Autodesk Inventor part; units mm, degrees
ref_plane "YZ Plane" through (0, 0, 0) normal (1, 0, 0) x (0, 1, 0)
ref_plane "XZ Plane" through (0, 0, 0) normal (0, 1, 0) x (-1, 0, 0)
ref_plane "XY Plane" through (0, 0, 0) normal (0, 0, 1) x (1, 0, 0)
sketch "Эскиз1" plane through (0, 0, 0) normal (0, 0, 1) x (1, 0, 0)
  line L0 (0, 0) -> (0, 13)
  line L1 (0, 13) -> (16.5, 13)
  line L2 (16.5, 13) -> (16.5, 10)
  line L3 (16.5, 10) -> (14.5, 10)
  line L4 (14.5, 10) -> (14.5, 3)
  line L5 (14.5, 3) -> (13.5, 3)
  line L6 (13.5, 3) -> (13.5, 0)
  line L7 (13.5, 0) -> (0, 0)
  dimension "d0" = 13
  dimension "d1" = 16.5
  dimension "d2" = 3
  dimension "d3" = 2
  dimension "d4" = 7
  dimension "d5" = 1
revolve "Вращение1" add sketch "Эскиз1" angle 360 about axis through (0, 0, 0) along (0, 1, 0)
sketch "Эскиз2" plane through (0, 13, 0) normal (0, 1, 0) x (1, 0, 0)
  circle A0 centre (0, 0) radius 3
  line L0 (-5, -7) -> (5, -7)
  line L1 (7, -5) -> (7, 5)
  line L2 (5, 7) -> (-5, 7)
  line L3 (-7, 5) -> (-7, -5)
  line L4 (-7, -7) -> (7, 7) construction
  line L5 (7, -7) -> (-7, 7) construction
  arc A1 (-7, -5) -> (-5, -7) centre (-5, -5) ccw
  arc A2 (5, -7) -> (7, -5) centre (5, -5) ccw
  arc A3 (7, 5) -> (5, 7) centre (5, 5) ccw
  arc A4 (-5, 7) -> (-7, 5) centre (-5, 5) ccw
  dimension "d7" = 6
  dimension "d8" = 14
  dimension "d9" = 14
  dimension "d10" = 2
extrude "Выдавливание1" cut sketch "Эскиз2" against normal blind 24 contours A0
extrude "Выдавливание2" add sketch "Эскиз2" along normal blind 5
chamfer "Фаска1" distance 2 angle 45 8 edges at (0, 13, 7) (-6.4142, 13, 6.4142) (-7, 13, 0) (-6.4142, 13, -6.4142) (0, 13, -7) (6.4142, 13, -6.4142) (7, 13, 0) (6.4142, 13, 6.4142)
thread "Резьба1"
properties part number "Top_contact" material "Сталь нержавеющая AISI 202"
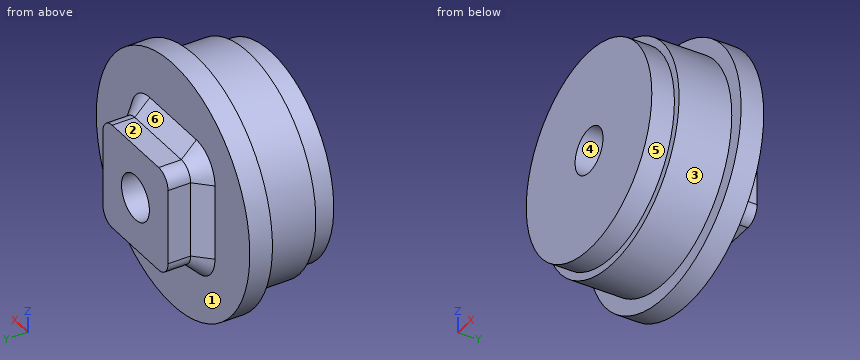
The model under review builds one solid part; all positions refer to its coordinate system, in mm. Face numbers are marked on the shaded views. A direction names the side the tool comes from. Give positions to 0.01 mm unless a question says otherwise; leave off trailing zeros. Write each loop counter-clockwise with the first axis right and the second up, starting at its lowest first coordinate (ties: lowest second). Pieces come first, ordered by that corner, then holes. Notation, with made-up numbers: M 5,78.5 L 31,78.5 A4 cw 31,83.5 Z; hole C 16,-10.75 d7. An arc over 180 degrees is marked long. Write each question's results on one line, items separated by ' | '. Start each with the question number.
1. We need section C-C (y = 14). Write out the cut boundary in (x, z), and give its area (3 significant figures).
2. Mouldability with a two-part tool opening along Z and no side actions: class the marked faces 4, 5 and 6 as released by +Z, released by -Z, zero draft, split by the parting line, or undercut.
3. We need section A-A (x = 0). Write out the cut boundary in (y, z).
4. Insertion check: pin 1 Ø2 at (x, y) = (-6, 13.5) entering from -Z; pin 2 Ø3 at (y, z) = (12, -7.5) entering from +X; pin 3 Ø2.5 at (x, y) = (2, 17) entering from -Z. Each pin has a flat end and moves straight along its axis. Give the tip position at first contact, or say it passes through.
5. For probe 1 along X at (y, z) = (11.5, 0); probe 2 along X at (y, z) = (17, -4), list the stretches that pass through material, from the lowest coordinate up. Write a range as [from, to].
6. For the marked faces 1, 2 and 3, list the 3-axis set-ups (+Z, -Z, +X, -X, +Y, -Y) from which the entire face can be reached by the end or side of a thin tool; tool diameter is ignored.
7. We need section B-B (z = 0). Write out the cut boundary in (x, y).
8. We need section D-D (z = 4). Write out the cut boundary in (x, y).
Results found:
1) outline: M -8,-5 A3 ccw -5,-8 L 5,-8 A3 ccw 8,-5 L 8,5 A3 ccw 5,8 L -5,8 A3 ccw -8,5 Z; hole C 0,0 d6 | area: 220 mm^2
2) face 4: undercut | face 5: split by the parting line | face 6: released by +Z
3) outline: M 0,-13.5 L 3,-13.5 L 3,-14.5 L 10,-14.5 L 10,-16.5 L 13,-16.5 L 13,-9 L 15,-7 L 18,-7 L 18,-3 L 0,-3 Z; M 0,3 L 18,3 L 18,7 L 15,7 L 13,9 L 13,16.5 L 10,16.5 L 10,14.5 L 3,14.5 L 3,13.5 L 0,13.5 Z
4) pin 1: stops at z = -15.68 | pin 2: stops at x = 15.37 | pin 3: stops at z = -7
5) probe 1: x = [-16.5, -3], [3, 16.5] | probe 2: x = [-7, 7]
6) face 1: +Y | face 2: +Z, +X, -X, +Y | face 3: -Y
7) outline: M -16.5,10 L -14.5,10 L -14.5,3 L -13.5,3 L -13.5,0 L -3,0 L -3,18 L -7,18 L -7,15 L -9,13 L -16.5,13 Z; M 3,0 L 13.5,0 L 13.5,3 L 14.5,3 L 14.5,10 L 16.5,10 L 16.5,13 L 9,13 L 7,15 L 7,18 L 3,18 Z
8) outline: M -16.01,10 L -13.94,10 L -13.94,3 L -12.89,3 L -12.89,0 L 12.89,0 L 12.89,3 L 13.94,3 L 13.94,10 L 16.01,10 L 16.01,13 L 9,13 L 7,15 L 7,18 L -7,18 L -7,15 L -9,13 L -16.01,13 Z
